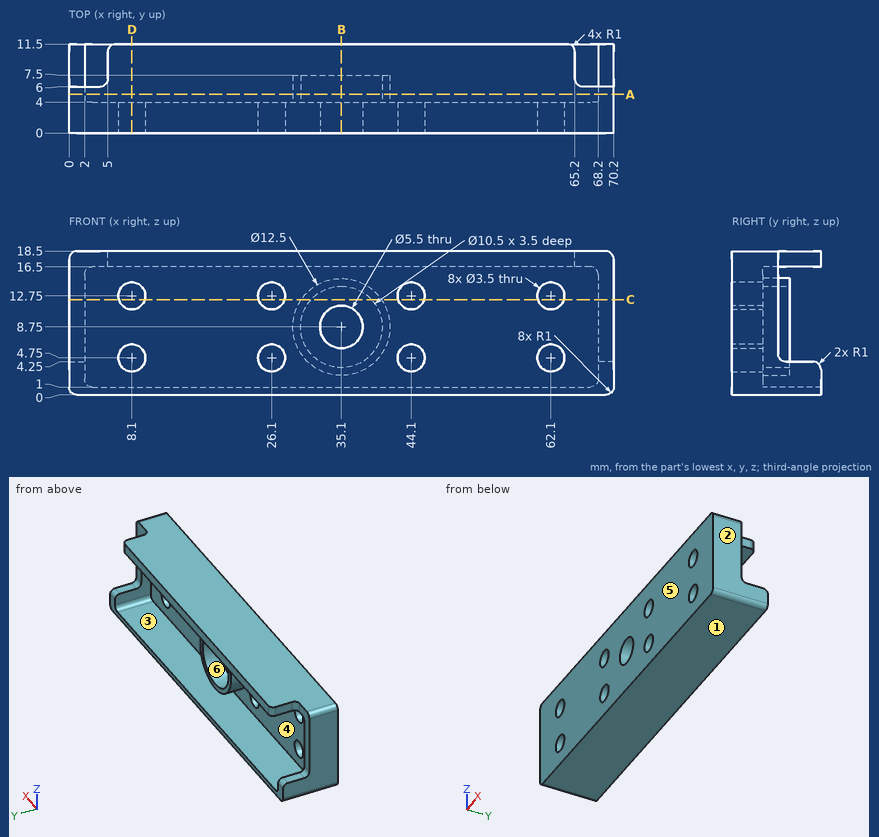
Source: three-view drawing plus pictorial views. Frame: mm from the lowest corner of the part. A direction names the side the tool comes from. Round coordinates to 2 decimals unless told otherwise and drop trailing zeros. Loops run counter-clockwise (first coordinate to the right, second up) from the corner with the lowest first, then second, coordinate; pieces in that order, holes last.
Q1. Ray query, line 1 (Z direction, x = 26.1, y = 0.9); line 2 (X direction, y = 2.75, z = 12.75); line 3 (Z direction, x = 35.1, y = 1.1). Return the intervals inside material, ascending.
Q2. Mould query, pull axis Z, two halves, no side actions, for the marked faces 1, 2, 3 and 4. Classes: pulls with the +Z half, pulls with the -Z half, needs draft (parallel to the pull), parting line crosses it, or undercut.
Q3. First-contact query: P1, Ø3, axis at x = 62.1, z = 4.75, coming from the +Y side; P2, Ø5, axis at y = 7, z = 15.5, coming from the +X side; P3, Ø1, axis at x = 0.5, y = 8.5, coming from the +Z side; P4, Ø4.5, axis at x = 68, z = 13.5, coming from the +Y side. Flat tips, straight axial feed; report the tip coordinate or a pass-through.
Q4. Section D-D, the plane x = 8.1. Return loops of the section in (y, z), plus the area to 3 significant figures.
Q5. Section C-C, the plane z = 12.25. State how many separate pieces and enclosed holes the cut face has, plus the area to 3 significant figures.
Q6. Section A-A, the plane y = 5. Return loops of the section in (x, z), plus the area to 3 significant figures.
Q7. Section B-B, the plane x = 35.1. Return loops of the section in (y, z), plus the area to 3 significant figures.
Q8. Access query for the marked faces 5 and 6. Directions: +Z, -Z, +X, -X, +Y, -Y. A direction counts if a zero-diameter tool reaches every point of the face in a straight line with its end or side. Return the directions, or none.
Solutions:
1. line 1: z = 0 to 3, 6.5 to 11, 14.5 to 18.5
1. line 2: x = 0 to 6.35, 9.85 to 24.35, 27.85 to 42.35, 45.85 to 60.35, 63.85 to 70.2
1. line 3: z = 0 to 6, 11.5 to 18.5
2. face 1: pulls with the -Z half
2. face 2: needs draft
2. face 3: undercut
2. face 4: undercut
3. P1: passes through
3. P2: stops at x = 70.2
3. P3: stops at z = 4.25
3. P4: stops at y = 6
4. outline: (0, 0) - (11.5, 0) - (11.5, 1) - (4, 1) - (4, 3) - (0, 3) - close; (0, 6.5) - (4, 6.5) - (4, 11) - (0, 11) - close; (0, 14.5) - (4, 14.5) - (4, 16.5) - (11.5, 16.5) - (11.5, 18.5) - (0, 18.5) - close
4. area: 68.5 mm2
5. separate pieces: 5
5. enclosed holes: 0
5. area: 244 mm2
6. outline: (0, 1) arc R1 ccw to (1, 0) - (69.2, 0) arc R1 ccw to (70.2, 1) - (70.2, 17.5) arc R1 ccw to (69.2, 18.5) - (1, 18.5) arc R1 ccw to (0, 17.5) - close; circle Ø12.5 at (35.1, 8.75); hole (2, 2) arc R1 ccw to (3, 1) - (67.2, 1) arc R1 ccw to (68.2, 2) - (68.2, 15.5) arc R1 ccw to (67.2, 16.5) - (3, 16.5) arc R1 ccw to (2, 15.5) - close; hole circle Ø10.5 at (35.1, 8.75)
6. area: 309 mm2
7. outline: (0, 0) - (11.5, 0) - (11.5, 1) - (4, 1) - (4, 2.5) - (7.5, 2.5) - (7.5, 3.5) - (4, 3.5) - (4, 6) - (0, 6) - close; (0, 11.5) - (4, 11.5) - (4, 14) - (7.5, 14) - (7.5, 15) - (4, 15) - (4, 16.5) - (11.5, 16.5) - (11.5, 18.5) - (0, 18.5) - close
7. area: 81.5 mm2
8. face 5: +Z, -Z, +X, -X, -Y
8. face 6: +Y
